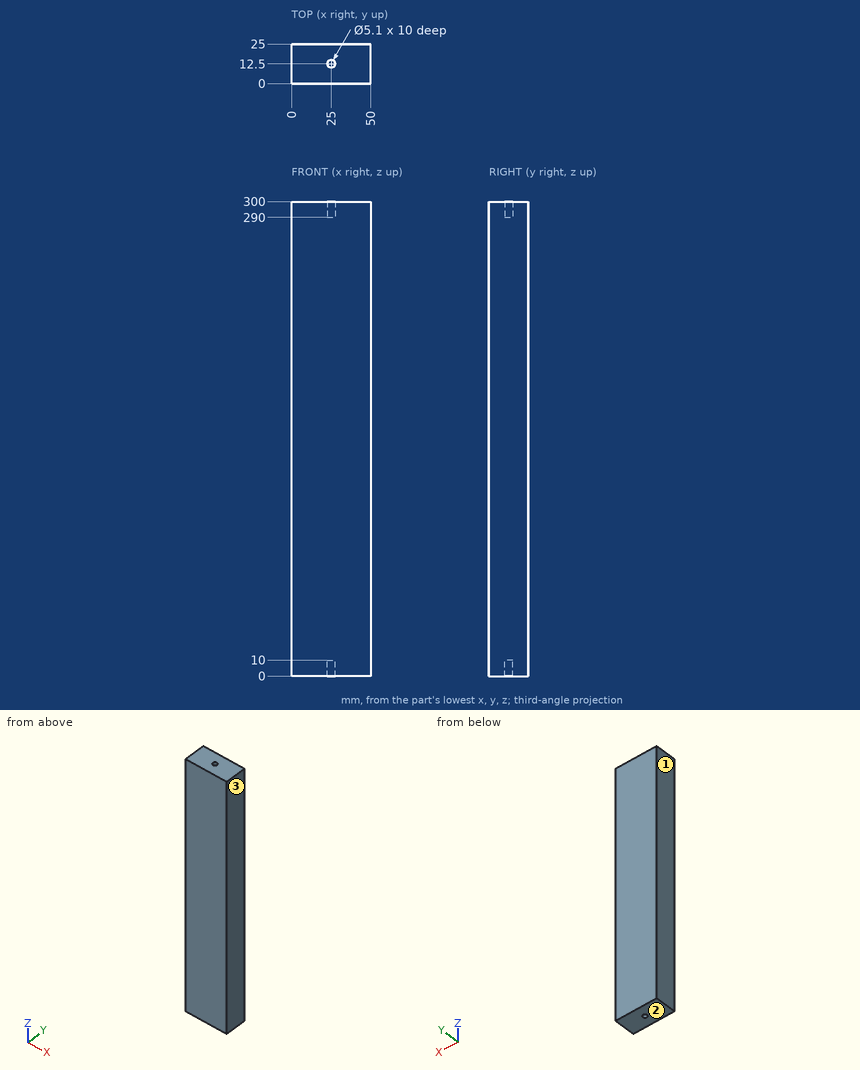
Geometry check sheet. Reference: drawing and pictorial views, mm from the part's lowest x, y, z. Round coordinates to 2 decimals unless told otherwise and drop trailing zeros. One line per item, written item: value. Start each with the question number.
Q1. Thickness scan on line 1 (X direction, y = 12.5, z = 293.5); line 2 (Y direction, x = 25, z = 293.75). Record the ranges inside material, lowest first.
Q2. Mould release check, pull along X, two halves, no side actions. Record for the marked faces 1, 2 and 3: pulls with the +X half, pulls with the -X half, needs draft (parallel to the pull), parting line crosses it, or undercut.
Q3. Gauge pin test, flat ends, axial feed: pin 1 Ø1.5 at (x, y) = (25, 12) entering from +Z; pin 2 Ø4.5 at (x, y) = (25, 12.5) entering from -Z. Record the tip position at first contact, or that the pin passes through.
Completed:
1. line 1: x = 0 to 22.45, 27.55 to 50
1. line 2: y = 0 to 9.95, 15.05 to 25
2. face 1: pulls with the -X half
2. face 2: needs draft
2. face 3: pulls with the +X half
3. pin 1: stops at z = 290
3. pin 2: stops at z = 10
